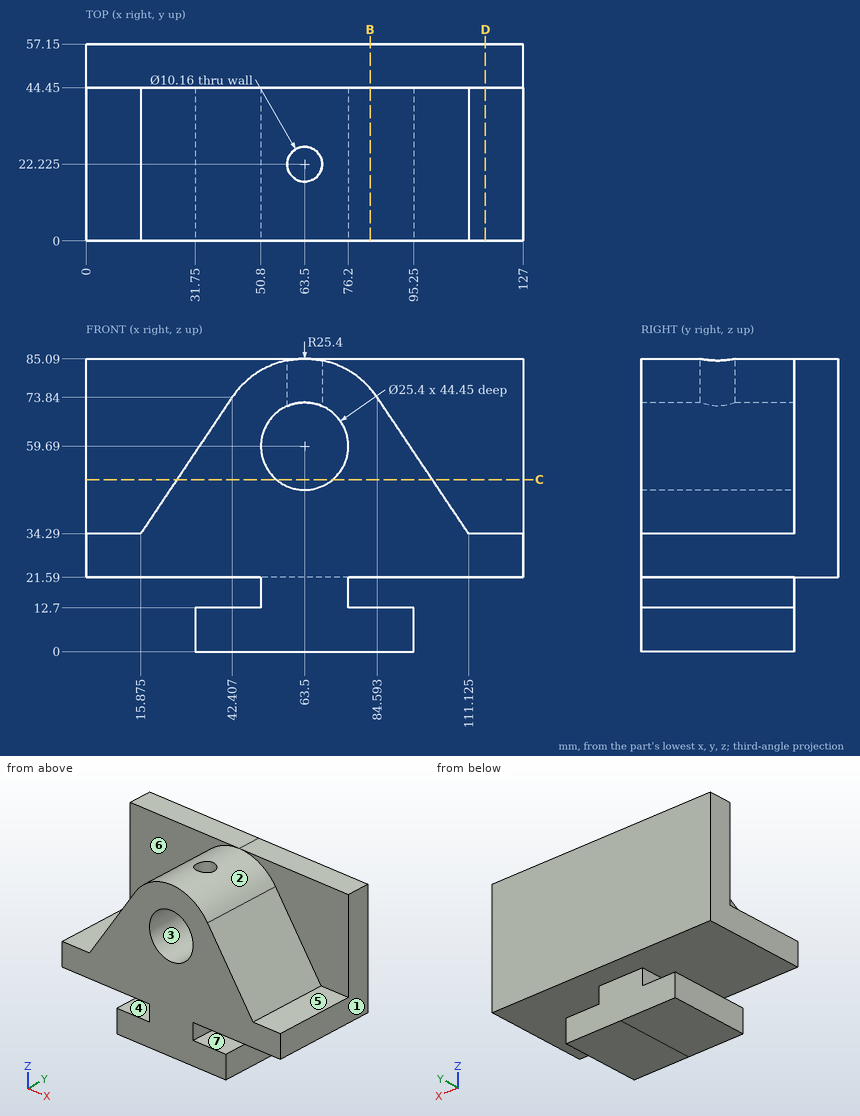
The drawing under review shows one solid part. Ordinate dimensions are in mm from its lowest x, y, z. A direction names the side the tool comes from. Round coordinates to 2 decimals unless told otherwise and drop trailing zeros. Write each loop counter-clockwise with the first axis right and the second up, starting at its lowest first coordinate (ties: lowest second). Pieces come first, ordered by that corner, then holes.
(1) Machinability: for the marked faces 4, 5, 6 and 7, which of the approach directions +Z, -Z, +X, -X, +Y, -Y give a long, thin tool a straight path to every point of the face, cutting with its end or side? Answer none if there is none.
(2) We need section D-D on x = 116. Give the boundary of the cut face in (y, z).
(3) Insertion check: pin 1 (15 mm diameter, centred on x = 81.5, y = 25, fed in from +Z); pin 2 (2 mm diameter, centred on x = 89, y = 51, fed in from -Z); pin 3 (2.5 mm diameter, centred on y = 18, z = 17.5, fed in from +X). Each pin has a flat end and moves straight along its axis. Give the tip position at first contact, or say it passes through.
(4) We need section C-C on z = 50. Give the boundary of the cut face in (x, y).
(5) Wall thickness on L1, parallel to X at y = 34, z = 14.5; L2, parallel to Y at x = 121, z = 60; L3, parallel to X at y = 29, z = 60.5 (1 decimal): over which ranges is each line inside the solid? List them lowest first.
(6) We need section B-B on x = 82.5. Give the boundary of the cut face in (y, z).
(7) Mouldability with a two-part tool opening along Z and no side actions: class the marked faces 1, 2 and 3 as +Z half, -Z half, draft (parallel to the pull), parting line (faces both ways), or undercut.
Findings below:
1. face 4: -X, +Y, -Y
1. face 5: +Z, +X, -Y
1. face 6: +Z, -X, -Y
1. face 7: +X, +Y, -Y
2. outline: (0, 21.59) - (57.15, 21.59) - (57.15, 85.09) - (44.45, 85.09) - (44.45, 34.29) - (0, 34.29) - close
3. pin 1: stops at z = 82.82
3. pin 2: stops at z = 21.59
3. pin 3: stops at x = 76.2
4. outline: (0, 44.45) - (26.41, 44.45) - (26.41, 0) - (55.29, 0) - (55.29, 44.45) - (71.71, 44.45) - (71.71, 0) - (100.59, 0) - (100.59, 44.45) - (127, 44.45) - (127, 57.15) - (0, 57.15) - close
5. L1: x = 50.8 to 76.2
5. L2: y = 44.45 to 57.15
5. L3: x = 33.5 to 50.8, 76.2 to 93.5
6. outline: (0, 0) - (44.45, 0) - (44.45, 12.7) - (0, 12.7) - close; (0, 21.59) - (57.15, 21.59) - (57.15, 85.09) - (44.45, 85.09) - (44.45, 76.55) - (0, 76.55) - close
7. face 1: draft
7. face 2: +Z half
7. face 3: undercut
